from build123d import *

# Parameters (mm, degrees)
SKETCH_1_W             = 160
SKETCH_1_H             = 15
EXTRUDE_1_DEPTH        = 10
HOLE_WIZARD_M5_1_D     = 4.2
HOLE_WIZARD_M5_1_DEPTH = 13
HOLE_WIZARD_M5_1_TIP   = 1.2618073
CHAMFER_1_SIZE         = 5
CUT_EXTRUDE_1_DEPTH    = 10


with BuildPart() as part:
    # 草图1 → 凸台-拉伸1 (new body)
    with BuildSketch(Plane.XY):
        with Locations((80, 7.5)):
            Rectangle(SKETCH_1_W, SKETCH_1_H)
    extrude(amount=EXTRUDE_1_DEPTH)

    # M5 螺纹孔1
    with Locations(Plane(origin=(7.5, 15, 5), x_dir=(0, 0, 1), z_dir=(0, 1, 0))):
        with Locations((0, 0), (0, 15)):
            Hole(HOLE_WIZARD_M5_1_D / 2, depth=HOLE_WIZARD_M5_1_DEPTH)
            with Locations((0, 0, -(HOLE_WIZARD_M5_1_DEPTH + HOLE_WIZARD_M5_1_TIP / 2))):  # 118° drill point
                Cone(0, HOLE_WIZARD_M5_1_D / 2, HOLE_WIZARD_M5_1_TIP, mode=Mode.SUBTRACT)

    # 倒角1
    chamfer_1_edges = [part.edges().sort_by_distance(p)[0] for p in [
        (0, 0, 5),
    ]]
    chamfer(chamfer_1_edges, length=CHAMFER_1_SIZE)

    # 草图4 → 切除-拉伸1 (cut)
    with BuildSketch(Plane(origin=(0, 0, 0), x_dir=(-1, 0, 0), z_dir=(0, 0, -1))):
        with BuildLine():
            Line((-152.5, 10.75), (-142.5, 10.75))
            ThreePointArc((-142.5, 10.75), (-139.25, 7.5), (-142.5, 4.25))
            Line((-142.5, 4.25), (-152.5, 4.25))
            ThreePointArc((-152.5, 4.25), (-155.75, 7.5), (-152.5, 10.75))
        make_face()
        with BuildLine():
            Line((-117.5, 10.75), (-107.5, 10.75))
            ThreePointArc((-107.5, 10.75), (-104.25, 7.5), (-107.5, 4.25))
            Line((-107.5, 4.25), (-117.5, 4.25))
            ThreePointArc((-117.5, 4.25), (-120.75, 7.5), (-117.5, 10.75))
        make_face()
    extrude(amount=-CUT_EXTRUDE_1_DEPTH, mode=Mode.SUBTRACT)


solid = part.part
Could you check a few things on this model? Use its own coordinates, in mm. A direction names the side the tool comes from. Give positions to 0.01 mm unless a question says otherwise; leave off trailing zeros. Order: outer loops, then holes, each group sorted by start corner. A loop starts at its lowest first (then second) coordinate and runs counter-clockwise, first axis right, second up.
Item 1: I need wall thicknesses on line 1 (X direction, y = 7.5, z = 5); line 2 (Z direction, x = 22.5, y = 6.25); line 3 (Y direction, x = 114, z = 2.25). Which ranges of each line are inside material? Lowest first, please.
Item 2: If we section it at B-B, the plane z = 8.5: Write out the boundary of the cut face in (x, y).
Item 3: For faces 1 (the face through (160, 7, 5)), 2 (the face through (9.582, 8.409, 5.273)), 3 (the face through (148, 10.75, 5)), which set-ups out of +Z, -Z, +X, -X, +Y, -Y let a thin tool reach every point of the face, with its end or its side?
Item 4: I'm going to push a flat-ended pin straight in: pin 1 (2 mm diameter, centred on y = 2, z = 4.5, fed in from -X). Where does the tip first touch, or does it pass through?
Item 5: If we mould it in two halves opening along Y, with no side actions, what happens to faces 4 (the face through (155.75, 7.43, 4.93)), 5 (the face through (79, 15, 5)), 6 (the face through (3, 2, 5))? For each: pulls with the +Y half, pulls with the -Y half, needs draft (parallel to the pull), parting line crosses it, or undercut.
Item 6: If we section it at A-A, the plane y = 7.5: Write out the boundary of the cut face in (x, z), plus the area to 3 significant figures.
Values:
1. line 1: x = 0 to 5.4, 9.6 to 20.4, 24.6 to 104.25, 120.75 to 139.25, 155.75 to 160
1. line 2: z = 0 to 2.9, 7.1 to 10
1. line 3: y = 0 to 4.25, 10.75 to 15
2. outline: (0, 5) - (5, 0) - (160, 0) - (160, 15) - (0, 15) - close; hole (107.5, 4.25) - (117.5, 4.25) arc R3.25 ccw to (117.5, 10.75) - (107.5, 10.75) arc R3.25 ccw to start; hole (142.5, 4.25) - (152.5, 4.25) arc R3.25 ccw to (152.5, 10.75) - (142.5, 10.75) arc R3.25 ccw to start
3. face 1: +Z, -Z, +X, +Y, -Y
3. face 2: +Y
3. face 3: +Z, -Z
4. pin 1: stops at x = 2
5. face 4: undercut
5. face 5: pulls with the +Y half
5. face 6: pulls with the -Y half
6. outline: (0, 0) - (104.25, 0) - (104.25, 10) - (0, 10) - close; (120.75, 0) - (139.25, 0) - (139.25, 10) - (120.75, 10) - close; (155.75, 0) - (160, 0) - (160, 10) - (155.75, 10) - close; hole circle Ø4.2 at (7.5, 5); hole circle Ø4.2 at (22.5, 5)
6. area: 1,240 mm2
